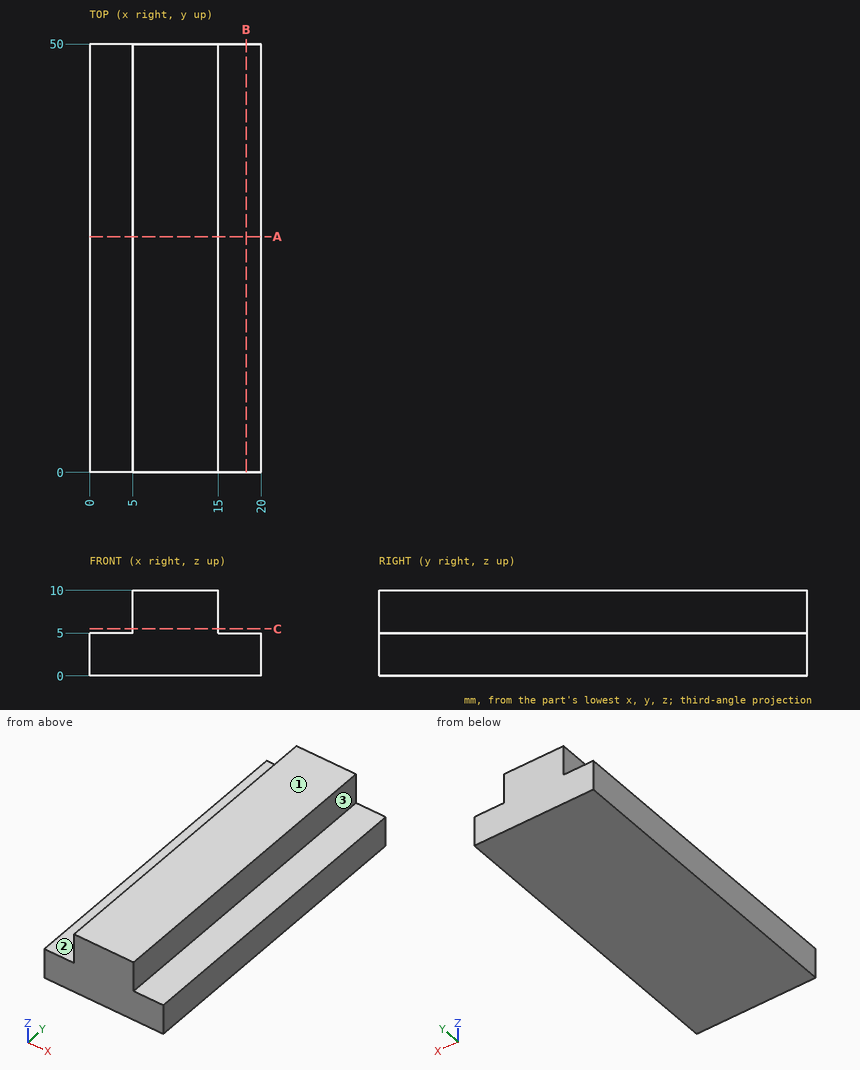
Could you check a few things on this drawing? It's one solid part, dimensions in mm from its lowest x, y, z. A direction names the side the tool comes from. Round coordinates to 2 decimals unless told otherwise and drop trailing zeros. Write each loop counter-clockwise with the first axis right and the second up, starting at its lowest first coordinate (ties: lowest second). Pieces come first, ordered by that corner, then holes. Notation, with made-up numbers: (89.25, 21.5) -> (100.25, 21.5) arc R19 cw to (100.25, 50.5) -> close; hole circle Ø9 at (85, 53). An arc over 180 degrees is marked (long way). One line per question, with ' | ' between items. Start each with the question number.
1) Suppose I cut it at B-B on x = 18.25. Write out the boundary of the cut face in (y, z).
2) Suppose I cut it at A-A on y = 27.5. Write out the boundary of the cut face in (x, z), then the cut area to 3 significant figures.
3) I'm going to push flat-ended pins straight in: P1, Ø4, axis at y = 34.5, z = 8.5, coming from the +X side; P2, Ø1.5, axis at x = 18, y = 27, coming from the +Z side; P3, Ø1.5, axis at y = 32.5, z = 6.5, coming from the -X side. Where does each tip first touch, or does it pass through?
4) I need wall thicknesses on line 1 (Z direction, x = 4, y = 13.5); line 2 (X direction, y = 19, z = 8.25). Which ranges of each line are inside material? Lowest first, please. Write a range as [from, to].
5) Suppose I cut it at C-C on z = 5.5. Write out the boundary of the cut face in (x, y), then the cut area to 3 significant figures.
6) On a 3-axis mill with a long thin cutter (end or side, diameter ignored), from which of +Z, -Z, +X, -X, +Y, -Y can I reach the whole of each face in a straight line? I mean the marked faces 1, 2 and 3. Say none if no direction works.
Return value:
1) outline: (0, 0) -> (50, 0) -> (50, 5) -> (0, 5) -> close
2) outline: (0, 0) -> (20, 0) -> (20, 5) -> (15, 5) -> (15, 10) -> (5, 10) -> (5, 5) -> (0, 5) -> close | area: 150 mm2
3) P1: stops at x = 15 | P2: stops at z = 5 | P3: stops at x = 5
4) line 1: z = [0, 5] | line 2: x = [5, 15]
5) outline: (5, 0) -> (15, 0) -> (15, 50) -> (5, 50) -> close | area: 500 mm2
6) face 1: +Z, +X, -X, +Y, -Y | face 2: +Z, -X, +Y, -Y | face 3: +Z, +X, +Y, -Y
